CAD build for the part. Positions are in the model's coordinates, mm. Face numbers are marked on the shaded views. A direction names the side the tool comes from. Give positions to 0.01 mm unless a question says otherwise; leave off trailing zeros. Loops run counter-clockwise (first coordinate to the right, second up) from the corner with the lowest first, then second, coordinate; pieces in that order, holes last. Notation, with made-up numbers: M 54.25,-14 L 97.25,-14 A19 ccw 97.25,-3 Z; hole C 72,26 d10. An arc over 180 degrees is marked long. Answer as CSV lines item,"result".
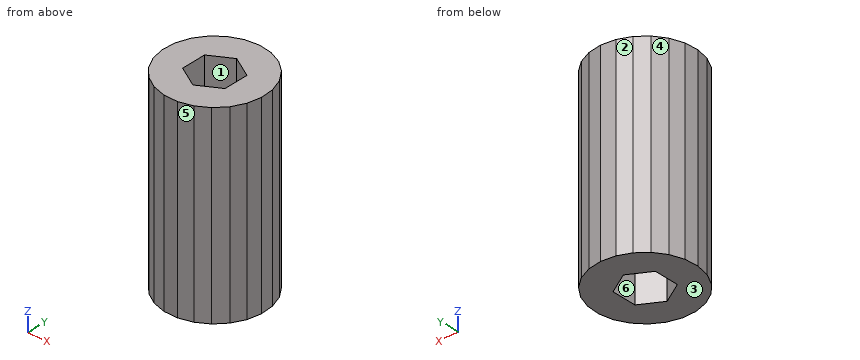
```python
from build123d import *

# Parameters (mm, degrees)
PAD_DEPTH = 25


with BuildPart() as part:
    # Sketch → Pad (new body)
    with BuildSketch(Plane.XY):
        Polygon((4.750434, 4.436595), (3.377296, 5.553726), (1.753679, 6.258962), (0, 6.5), (-1.753679, 6.258962), (-3.377296, 5.553726), (-4.750434, 4.436595), (-5.771254, 2.990423), (-6.364047, 1.322464), (-6.484847, -0.443576), (-6.124696, -2.176717), (-5.310304, -3.748422), (-4.102072, -5.042123), (-2.589607, -5.961873), (-0.885083, -6.439459), (0.885083, -6.439459), (2.589607, -5.961873), (4.102072, -5.042123), (5.310304, -3.748422), (6.124696, -2.176717), (6.484847, -0.443576), (6.364047, 1.322464), (5.771254, 2.990423), align=None)
        Polygon((2.771281, -1.6), (2.771281, 1.6), (0, 3.2), (-2.771281, 1.6), (-2.771281, -1.6), (0, -3.2), align=None, mode=Mode.SUBTRACT)
    extrude(amount=PAD_DEPTH)


solid = part.part
```
Q1. Wall check: line 1 (X direction, y = -0.25, z = 6); line 2 (X direction, y = -2, z = 16.5); line 3 (Y direction, x = 0.5, z = 16.75). Give the ranges that are in metal, low to high. Write a range as [from, to].
Solution:
line 1,"x = [-6.47, -2.77], [2.77, 6.47]"
line 2,"x = [-6.16, -2.08], [2.08, 6.16]"
line 3,"y = [-6.44, -2.91], [2.91, 6.43]"
Q2. Cut at D-D (y = -4.75). Write the cut outline in (x, z), and give its area (3 significant figures).
Solution:
outline,"M -4.37,0 L 4.37,0 L 4.37,25 L -4.37,25 Z"
area,"219 mm²"
Q3. Cut at B-B (y = 1). Write the cut outline in (x, z).
Solution:
outline,"M -6.39,0 L -2.77,0 L -2.77,25 L -6.39,25 Z; M 2.77,0 L 6.39,0 L 6.39,25 L 2.77,25 Z"
Q4. Cut at C-C (x = 0.25). Write the cut outline in (y, z).
Solution:
outline,"M -6.44,0 L -3.06,0 L -3.06,25 L -6.44,25 Z; M 3.06,0 L 6.47,0 L 6.47,25 L 3.06,25 Z"
Q5. Pin check, flat tips, straight feed: P1, Ø1, axis at x = 1, z = 4.5, coming from the +Y side; P2, Ø4, axis at y = 4.5, z = 12, coming from the -X side; P3, Ø1.5, axis at y = -2.5, z = 17, coming from the -X side. Stop position of each tip, or through.
Solution:
P1,"stops at y = 6.43"
P2,"stops at x = -5.95"
P3,"stops at x = -6.21"
Q6. Which spindle directions (+Z, -Z, +X, -X, +Y, -Y) get a long thin tool onto all of the face, cutting with end or side? Do the marked faces 1 and 2. Say none if no direction does.
Solution:
face 1,"+Z, -Z"
face 2,"+Z, -Z, -X, +Y"
Q7. Mould opens along X. For the marked faces 3, 4, 5 and 6 say: released by +X, released by -X, zero draft, split by the parting line, or undercut.
Solution:
face 3,"zero draft"
face 4,"released by -X"
face 5,"released by +X"
face 6,"undercut"
